```python
from build123d import *

# Parameters (mm, degrees)
SKETCH_1_R      = 6.579
SKETCH_1_R_2    = 4.25
EXTRUDE_1_DEPTH = 6
EXTRUDE_START   = 6
SKETCH_1_3_R    = 4.25
EXTRUDE_2_DEPTH = 6
SKETCH_2_R      = 6.579
SKETCH_2_R_2    = 5.079
EXTRUDE_3_DEPTH = 6


with BuildPart() as part:
    # Sketch 1 → Extrude 1 (new body)
    with BuildSketch(Plane(origin=(0, 0, 0), x_dir=(1, 0, 0), z_dir=(0, 1, 0))):
        with Locations(Location((0, 0, 0), (0, 0, 270))):
            Circle(SKETCH_1_R)
        with Locations(Location((0, 0, 0), (0, 0, 270))):
            Circle(SKETCH_1_R_2, mode=Mode.SUBTRACT)
    extrude(amount=-EXTRUDE_1_DEPTH)

    # Sketch 1_3 → Extrude 2 (add)
    with BuildSketch(Plane(origin=(0, 0, 0), x_dir=(1, 0, 0), z_dir=(0, 1, 0)).offset(EXTRUDE_START)):
        Polygon((-4.37573769, -7.579), (4.37573769, -7.579), (8.75147538, 0), (4.37573769, 7.579), (-4.37573769, 7.579), (-8.75147538, 0), align=None)
        with Locations(Location((0, 0, 0), (0, 0, 270))):
            Circle(SKETCH_1_3_R, mode=Mode.SUBTRACT)
    extrude(amount=-EXTRUDE_2_DEPTH)

    # Sketch 2 → Extrude 3 (add)
    with BuildSketch(Plane(origin=(0, 6, 0), x_dir=(1, 0, 0), z_dir=(0, 1, 0)).offset(EXTRUDE_START)):
        with Locations(Location((0, 0, 0), (0, 0, 270))):
            Circle(SKETCH_2_R)
        with Locations(Location((0, 0, 0), (0, 0, 270))):
            Circle(SKETCH_2_R_2, mode=Mode.SUBTRACT)
    extrude(amount=-EXTRUDE_3_DEPTH)


solid = part.part
```
Geometry: final body of the model. Coordinates: model frame, mm. A direction names the side the tool comes from. Round coordinates to 2 decimals unless told otherwise and drop trailing zeros. Write each loop counter-clockwise with the first axis right and the second up, starting at its lowest first coordinate (ties: lowest second). Pieces come first, ordered by that corner, then holes.
Item 1: Section query B-B (y = 2.25). Return loops of the section in (x, z), plus the area to 3 significant figures.
Item 2: Section query C-C (z = 2.25). Return loops of the section in (x, y), plus the area to 3 significant figures.
Item 3: Section query D-D (z = 6). Return loops of the section in (x, y), plus the area to 3 significant figures.
Item 4: Set-up query: faces 1 (the face through (5, 0, -5)), 2 (the face through (0, 3, -7.579)), 3 (the face through (2, 6, 4)). Return all of +Z, -Z, +X, -X, +Y, -Y with unobstructed straight access to the full face (end or side cutting, diameter ignored); none if empty.
Item 5: Mould query, pull axis X, two halves, no side actions, for faces 4 (the face through (-4.96, 9.04, -1.1)), 5 (the face through (-6.42, -2.96, -1.43)), 6 (the face through (-4.3, -6, 1.4)), 7 (the face through (-6.533, 3.042, -3.843)). Classes: +X half, -X half, draft (parallel to the pull), parting line (faces both ways), or undercut.
Item 6: Material intervals for L1, parallel to X at y = -1, z = 0; L2, parallel to X at y = 8.9, z = 0; L3, parallel to Y at x = -6, z = 4.25, sorted ascending.
Item 7: Pin query (flat end, axial travel): P1, Ø1.5, axis at y = -1.5, z = 3.5, coming from the -X side; P2, Ø4.5, axis at x = -0.5, z = 0.5, coming from the -Y side; P3, Ø2, axis at y = 5.5, z = -1.5, coming from the -X side; P4, Ø2, axis at y = 0.5, z = -5.5, coming from the +X side. Return the tip coordinate at first contact, or that it passes through.
Item 8: Section query A-A (x = 0). Return loops of the section in (y, z).
Completed:
1. outline: (-8.75, 0) - (-4.38, -7.58) - (4.38, -7.58) - (8.75, 0) - (4.38, 7.58) - (-4.38, 7.58) - close; hole circle Ø8.5 at (0, 0)
1. area: 142 mm2
2. outline: (-7.45, 0) - (-6.18, 0) - (-6.18, -6) - (-3.61, -6) - (-3.61, 6) - (-4.55, 6) - (-4.55, 12) - (-6.18, 12) - (-6.18, 6) - (-7.45, 6) - close; (3.61, -6) - (6.18, -6) - (6.18, 0) - (7.45, 0) - (7.45, 6) - (6.18, 6) - (6.18, 12) - (4.55, 12) - (4.55, 6) - (3.61, 6) - close
2. area: 96.6 mm2
3. outline: (-5.29, 0) - (-2.7, 0) - (-2.7, -6) - (2.7, -6) - (2.7, 0) - (5.29, 0) - (5.29, 6) - (2.7, 6) - (2.7, 12) - (-2.7, 12) - (-2.7, 6) - (-5.29, 6) - close
3. area: 128 mm2
4. face 1: -Y
4. face 2: -Z, +X, -X, +Y, -Y
4. face 3: +Y
5. face 4: undercut
5. face 5: parting line
5. face 6: draft
5. face 7: -X half
6. L1: x = -6.58 to -4.25, 4.25 to 6.58
6. L2: x = -6.58 to -5.08, 5.08 to 6.58
6. L3: y = 0 to 6
7. P1: stops at x = -5.98
7. P2: passes through
7. P3: stops at x = -8.46
7. P4: stops at x = 6.15
8. outline: (-6, -6.58) - (0, -6.58) - (0, -7.58) - (6, -7.58) - (6, -6.58) - (12, -6.58) - (12, -5.08) - (6, -5.08) - (6, -4.25) - (-6, -4.25) - close; (-6, 4.25) - (6, 4.25) - (6, 5.08) - (12, 5.08) - (12, 6.58) - (6, 6.58) - (6, 7.58) - (0, 7.58) - (0, 6.58) - (-6, 6.58) - close
